from build123d import *

# Parameters (mm, degrees)
F2_ANGLE = 30
F3_DEPTH = 25


with BuildPart() as f2:
    # F1 (on Right) → F2 (revolve)
    with BuildSketch(Plane.YZ):
        with BuildLine():
            Line((-55.786951, 12.00949), (-64.979339, 21.201879))
            ThreePointArc((-64.979339, 21.201879), (-66.458592, 19.571493), (-67.989844, 17.989844))
            Line((-67.989844, 17.989844), (-58.898221, 8.898221))
            Line((-58.898221, 8.898221), (-55.786951, 12.00949))
        make_face()
        with BuildLine():
            ThreePointArc((-67.989844, 17.989844), (-69.571493, 16.458592), (-71.201879, 14.979339))
            Line((-71.201879, 14.979339), (-62.00949, 5.786951))
            Line((-62.00949, 5.786951), (-58.898221, 8.898221))
            Line((-58.898221, 8.898221), (-67.989844, 17.989844))
        make_face()
    revolve(axis=Axis((0, 0, 12.074878), (0, 0, 1)), revolution_arc=F2_ANGLE)

    # F1 (on Right) → F3 (join)
    with BuildSketch(Plane.YZ):
        with BuildLine():
            ThreePointArc((-67.989844, 17.989844), (-69.571493, 16.458592), (-71.201879, 14.979339))
            Line((-71.201879, 14.979339), (-62.00949, 5.786951))
            Line((-62.00949, 5.786951), (-58.898221, 8.898221))
            Line((-58.898221, 8.898221), (-67.989844, 17.989844))
        make_face()
        with BuildLine():
            Line((-55.786951, 12.00949), (-64.979339, 21.201879))
            ThreePointArc((-64.979339, 21.201879), (-66.458592, 19.571493), (-67.989844, 17.989844))
            Line((-67.989844, 17.989844), (-58.898221, 8.898221))
            Line((-58.898221, 8.898221), (-55.786951, 12.00949))
        make_face()
    extrude(amount=-F3_DEPTH)


solid = f2.part
Here's how the part is built. I have some questions about the finished solid (model axes, mm). A direction names the side the tool comes from. Give positions to 0.01 mm unless a question says otherwise; leave off trailing zeros. Order: outer loops, then holes, each group sorted by start corner. A loop starts at its lowest first (then second) coordinate and runs counter-clockwise, first axis right, second up. Notation, with made-up numbers: M 0,8.5 L 45,8.5 A16 ccw 45,12.5 Z; hole C -4,78 d9. An arc over 180 degrees is marked long. Answer as a JSON object with one key per item and string values. Group by question number.
1) Suppose I cut it at B-B, the plane z = 10. Write out the boundary of the cut face in (x, y), plus the area to 3 significant figures.
2) Suppose I cut it at A-A, the plane x = -17.5. Write out the boundary of the cut face in (y, z).
3) On a 3-axis mill with a long thin cutter (end or side, diameter ignored), from which of +Z, -Z, +X, -X, +Y, -Y can I reach the whole of each face in a straight line? I mean faces 1 (the flat face through (-25, -64, 14)), 2 (the flat face through (-12.32, -60.32, 16.54)). Say none if no direction works.
4) I'm going to push flat-ended pins straight in: pin 1 Ø8 at (x, y) = (-18.5, -56.5) entering from +Z; pin 2 Ø6 at (x, z) = (14.5, 16) entering from +Y; pin 3 Ø5 at (x, y) = (-1.5, -58) entering from -Z; pin 4 Ø3 at (y, z) = (-51, 18.5) entering from +X. Where does each tip first touch, or does it pass through?
5) Please list where these lines run through material, in increasing order: L1, parallel to Y at x = 24, z = 13; L2, parallel to Y at x = 14, z = 7.5; L3, parallel to Z at x = 18, y = -62.5. Write a range as [from, to].
Results found:
{
 "1": {"outline": "M -25,-66.22 L 0,-66.22 A66.22 ccw 33.11,-57.35 L 28.9,-50.05 A57.8 cw 0,-57.8 L -25,-57.8 Z", "area": "484 mm²"},
 "2": {"outline": "M -71.2,14.98 L -62.01,5.79 L -58.9,8.9 L -55.79,12.01 L -64.98,21.2 A68 cw -67.99,17.99 A68 cw Z"},
 "3": {"face 1": "+Z, -Z, -X, +Y, -Y", "face 2": "+Z, -X, +Y"},
 "4": {"pin 1": "z = 16.72", "pin 2": "y = -54.79", "pin 3": "z = 7.3", "pin 4": "through"},
 "5": {"L1": "[-64.93, -51.46]", "L2": "[-62.17, -58.65]", "L3": "[8.82, 21.13]"}
}
